The drawing under review shows one solid part. Ordinate dimensions are in mm from its lowest x, y, z. A direction names the side the tool comes from. Coordinates: 2 decimals unless noted, no trailing zeros. Order: outer loops, then holes, each group sorted by start corner. A loop starts at its lowest first (then second) coordinate and runs counter-clockwise, first axis right, second up.
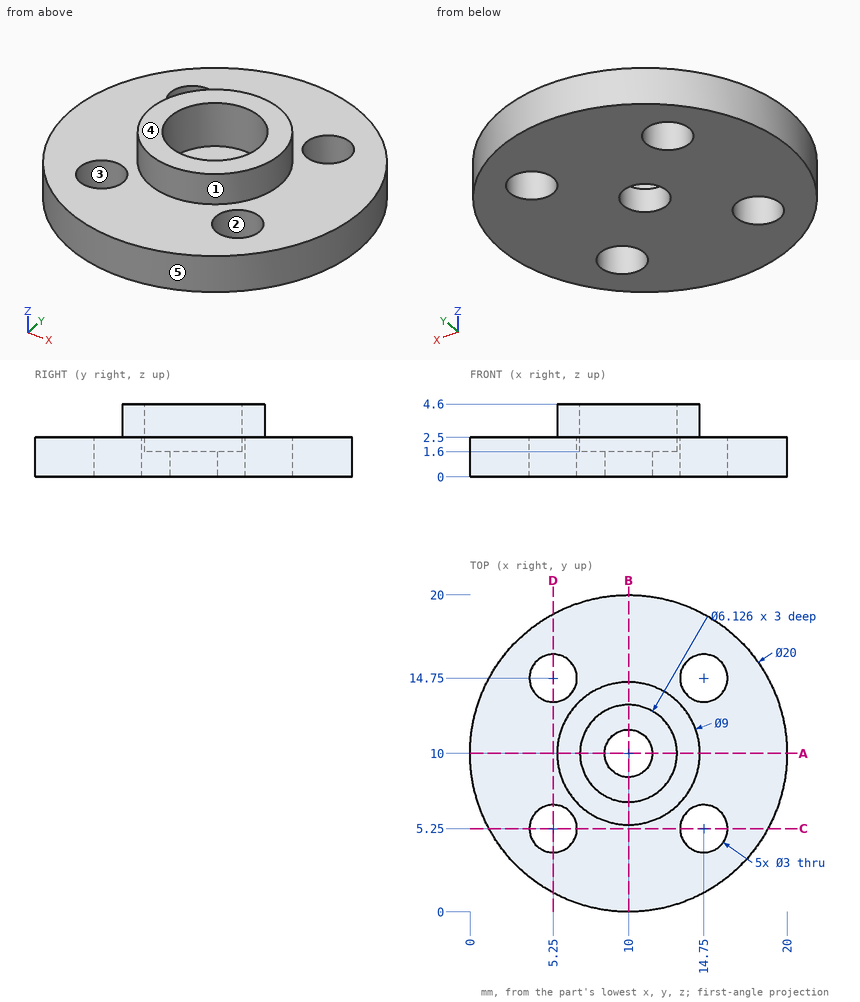
(1) Tool access review of the marked faces 1 and 2: name each direction out of +Z, -Z, +X, -X, +Y, -Y from which nothing blocks a thin tool from reaching the whole face with its end or side.
(2) Wall thickness on line 1 (Y direction, x = 14.75, z = 1.75); line 2 (Y direction, x = 10, z = 0.4); line 3 (Y direction, x = 15.75, z = 1.95): over which ranges is each line inside the solid? List them lowest first.
(3) Insertion check: pin 1 Ø5.5 at (x, y) = (10, 10) entering from +Z; pin 2 Ø2.5 at (x, y) = (5.25, 5.25) entering from -Z; pin 3 Ø2 at (x, z) = (8.5, 2.5) entering from +Y; pin 4 Ø1.5 at (x, z) = (13, 3.5) entering from +Y. Each pin has a flat end and moves straight along its axis. Give the tip position at first contact, or say it passes through.
(4) The part is to be moulded in two halves that separate along X. For the marked faces 3, 4 and 5, say which applies: +X half, -X half, draft (parallel to the pull), parting line (faces both ways), or undercut.
(5) Consider section A-A (y = 10). Give the boundary of the cut face in (x, z), then the cut area to 3 significant figures.
(6) Consider section C-C (y = 5.25). Give the boundary of the cut face in (x, z).
Findings:
1. face 1: +Z
1. face 2: +Z, -Z
2. line 1: y = 1.2 to 3.75, 6.75 to 13.25, 16.25 to 18.8
2. line 2: y = 0 to 8.5, 11.5 to 20
2. line 3: y = 1.82 to 4.13, 6.37 to 13.63, 15.87 to 18.18
3. pin 1: stops at z = 1.6
3. pin 2: passes through
3. pin 3: stops at y = 19.99
3. pin 4: stops at y = 13.9
4. face 3: undercut
4. face 4: draft
4. face 5: parting line
5. outline: (0, 0) - (8.5, 0) - (8.5, 1.6) - (6.94, 1.6) - (6.94, 4.6) - (5.5, 4.6) - (5.5, 2.5) - (0, 2.5) - close; (11.5, 0) - (20, 0) - (20, 2.5) - (14.5, 2.5) - (14.5, 4.6) - (13.06, 4.6) - (13.06, 1.6) - (11.5, 1.6) - close
5. area: 45.7 mm2
6. outline: (1.2, 0) - (3.75, 0) - (3.75, 2.5) - (1.2, 2.5) - close; (6.75, 0) - (13.25, 0) - (13.25, 2.5) - (6.75, 2.5) - close; (16.25, 0) - (18.8, 0) - (18.8, 2.5) - (16.25, 2.5) - close
